Work out the finished part from the listing and answer in its coordinate system (mm). Coordinates: 2 decimals unless noted, no trailing zeros. Answer as a JSON object with one key per item and string values. Group by question number.
1) Each of these flat-tipped pins is pushed along its axis until it touches: P1, Ø4, axis at x = 5.5, y = 13.5, coming from the +Z side; P2, Ø4.5, axis at x = 3, y = 8.5, coming from the +Z side; P3, Ø2, axis at x = 2.5, z = 14, coming from the -Y side. Where does it stop, or does it pass through?
2) Find the intervals of material crossed by line 1 along Y through (x, z) = (1.5, 6.5); line 2 along Z through (x, y) = (3, -7.5); line 3 along Y through (x, z) = (9, 8), in increasing order.
3) Section A-A (x = 9) is taken. Count the separate pieces of the cut face and the enclosed holes in it, plus the area to 3 significant figures.
from build123d import *

# Parameters (mm, degrees)
CUT_EXTRUDE2_DEPTH      = 30.467269979
FILLET1_R               = 0.75
CUT_EXTRUDE3_DEPTH      = 30.467269979
CUT_EXTRUDE3_DEPTH_BACK = 30.467269979
SKETCH2_R               = 1.5


with BuildPart() as part:
    # Sketch1 → Revolve2 (revolve)
    with BuildSketch(Plane.XY, mode=Mode.PRIVATE) as revolve2_sk:
        with BuildLine():
            Line((0, 0), (10, 0))
            Line((10, 0), (10, 19.6))
            Line((10, 19.6), (8.5, 19.6))
            ThreePointArc((8.5, 19.6), (5, 18.170714214), (1.5, 19.6))
            Line((1.5, 19.6), (0, 19.6))
            Line((0, 19.6), (0, 0))
        make_face()
    revolve(revolve2_sk.sketch.rotate(Axis((0, 0, 0), (1, 0, 0)), 90), axis=Axis((0, 0, 0), (1, 0, 0)))

    # Sketch3 → Cut-Extrude2 (cut, through all)
    with BuildSketch(Plane(origin=(10, 0, 0), x_dir=(0, 0, -1), z_dir=(1, 0, 0))):
        with BuildLine():
            Line((2.604722665, 14.772116295), (0.84225046, 4.776639722))
            ThreePointArc((0.84225046, 4.776639722), (1.566792192, 4.590297931), (2.25405939, 4.294751347))
            Line((2.25405939, 4.294751347), (6.970847581, 13.281840385))
            ThreePointArc((6.970847581, 13.281840385), (4.845422268, 14.195840343), (2.604722665, 14.772116295))
        make_face()
        with BuildLine():
            Line((9.171312121, 11.869584406), (2.965590908, 3.838091119))
            ThreePointArc((2.965590908, 3.838091119), (3.520543403, 3.336382325), (3.991740938, 2.755299829))
            Line((3.991740938, 2.755299829), (12.344757988, 8.520971201))
            ThreePointArc((12.344757988, 8.520971201), (10.887544298, 10.318012365), (9.171312121, 11.869584406))
        make_face()
        with BuildLine():
            Line((13.636864497, 6.247873773), (4.409550218, 2.020282094))
            ThreePointArc((4.409550218, 2.020282094), (4.667780547, 1.318141736), (4.814962743, 0.584642325))
            Line((4.814962743, 0.584642325), (14.890633111, 1.808050204))
            ThreePointArc((14.890633111, 1.808050204), (14.435461139, 4.076452099), (13.636864497, 6.247873773))
        make_face()
        with BuildLine():
            Line((14.978375558, -0.805149446), (4.843334715, -0.260349211))
            ThreePointArc((4.843334715, -0.260349211), (4.74568542, -1.002069239), (4.53513461, -1.719949689))
            Line((4.53513461, -1.719949689), (14.02524364, -5.319073306))
            ThreePointArc((14.02524364, -5.319073306), (14.676387798, -3.098974216), (14.978375558, -0.805149446))
        make_face()
        with BuildLine():
            Line((12.888521288, -7.67372263), (4.167569596, -2.48133765))
            ThreePointArc((4.167569596, -2.48133765), (3.736410956, -3.092718228), (3.216361792, -3.630521958))
            Line((3.216361792, -3.630521958), (9.946839874, -11.227661223))
            ThreePointArc((9.946839874, -11.227661223), (11.555130883, -9.564462885), (12.888521288, -7.67372263))
        make_face()
        with BuildLine():
            Line((7.846062115, -12.784338438), (2.537064508, -4.133881536))
            ThreePointArc((2.537064508, -4.133881536), (1.87116977, -4.474862742), (1.160759249, -4.709385399))
            Line((1.160759249, -4.709385399), (3.589734964, -14.564127261))
            ThreePointArc((3.589734964, -14.564127261), (5.786732737, -13.838848371), (7.846062115, -12.784338438))
        make_face()
        with BuildLine():
            ThreePointArc((0.325348516, -4.839402981), (-0.42273386, -4.83187013), (-1.160759249, -4.709385399))
            Line((-1.160759249, -4.709385399), (-3.589734964, -14.564127261))
            ThreePointArc((-3.589734964, -14.564127261), (-1.307336141, -14.942920471), (1.006164666, -14.966216378))
            Line((1.006164666, -14.966216378), (0.325348516, -4.839402981))
        make_face()
        with BuildLine():
            ThreePointArc((-1.9609009, -4.436275524), (-2.619794257, -4.081954301), (-3.216361792, -3.630521958))
            Line((-3.216361792, -3.630521958), (-9.946839874, -11.227661223))
            ThreePointArc((-9.946839874, -11.227661223), (-8.101910065, -12.623749574), (-6.064232982, -13.719514508))
            Line((-6.064232982, -13.719514508), (-1.9609009, -4.436275524))
        make_face()
        with BuildLine():
            ThreePointArc((-3.797931552, -3.016850808), (-4.216691362, -2.396911935), (-4.53513461, -1.719949689))
            Line((-4.53513461, -1.719949689), (-14.02524364, -5.319073306))
            ThreePointArc((-14.02524364, -5.319073306), (-13.040434031, -7.412629781), (-11.745387936, -9.329837203))
            Line((-11.745387936, -9.329837203), (-3.797931552, -3.016850808))
        make_face()
        with BuildLine():
            ThreePointArc((-4.764901855, -0.906301928), (-4.847595293, -0.162765931), (-4.814962743, 0.584642325))
            Line((-4.814962743, 0.584642325), (-14.890633111, 1.808050204))
            ThreePointArc((-14.890633111, 1.808050204), (-14.991551715, -0.503365838), (-14.735816061, -2.802806631))
            Line((-14.735816061, -2.802806631), (-4.764901855, -0.906301928))
        make_face()
        with BuildLine():
            ThreePointArc((-4.640290566, 1.411869801), (-4.367973561, 2.108667787), (-3.991740938, 2.755299829))
            Line((-3.991740938, 2.755299829), (-12.344757988, 8.520971201))
            ThreePointArc((-12.344757988, 8.520971201), (-13.508285569, 6.521213153), (-14.350446312, 4.366313163))
            Line((-14.350446312, 4.366313163), (-4.640290566, 1.411869801))
        make_face()
        with BuildLine():
            ThreePointArc((-3.45264463, 3.406599173), (-2.887701727, 3.897031127), (-2.25405939, 4.294751347))
            Line((-2.25405939, 4.294751347), (-6.970847581, 13.281840385))
            ThreePointArc((-6.970847581, 13.281840385), (-8.930433992, 12.051860799), (-10.677562255, 10.53516323))
            Line((-10.677562255, 10.53516323), (-3.45264463, 3.406599173))
        make_face()
        with BuildLine():
            ThreePointArc((-1.474039418, 4.620917729), (-0.745892228, 4.7926316), (0, 4.850327089))
            Line((0, 4.850327089), (0, 15))
            ThreePointArc((0, 15), (-2.30672761, 14.821572377), (-4.558577364, 14.290534364))
            Line((-4.558577364, 14.290534364), (-1.474039418, 4.620917729))
        make_face()
    extrude(amount=-CUT_EXTRUDE2_DEPTH, mode=Mode.SUBTRACT)

    # Fillet1
    fillet1_edges = [part.edges().sort_by_distance(p)[0] for p in [
        (5, -11.227661223, -9.946839874),
        (5, 2.755299829, -3.991740938),
        (5, 3.838091119, -2.965590908),
        (5, 11.869584406, -9.171312121),
        (5, 8.520971201, -12.344757988),
        (5, 0.584642325, -4.814962743),
        (5, 2.020282094, -4.409550218),
        (5, 6.247873773, -13.636864497),
        (5, 1.808050204, -14.890633111),
        (5, 4.294751347, 2.25405939),
        (5, 3.406599173, 3.45264463),
        (5, 10.53516323, 10.677562255),
        (5, 13.281840385, 6.970847581),
        (5, 4.850327089, 0),
        (5, 4.620917729, 1.474039418),
        (5, 14.290534364, 4.558577364),
        (5, 15, 0),
        (5, 0.584642325, 4.814962743),
        (5, -0.906301928, 4.764901855),
        (5, -2.802806631, 14.735816061),
        (5, 1.808050204, 14.890633111),
        (5, 2.755299829, 3.991740938),
        (5, 1.411869801, 4.640290566),
        (5, 4.366313163, 14.350446312),
        (5, 8.520971201, 12.344757988),
        (5, 4.294751347, -2.25405939),
        (5, 4.776639722, -0.84225046),
        (5, 14.772116295, -2.604722665),
        (5, 13.281840385, -6.970847581),
        (5, -4.709385399, -1.160759249),
        (5, -4.133881536, -2.537064508),
        (5, -12.784338438, -7.846062115),
        (5, -14.564127261, -3.589734964),
        (5, -4.709385399, 1.160759249),
        (5, -4.839402981, -0.325348516),
        (5, -14.966216378, -1.006164666),
        (5, -14.564127261, 3.589734964),
        (5, -1.719949689, 4.53513461),
        (5, -3.016850808, 3.797931552),
        (5, -9.329837203, 11.745387936),
        (5, -5.319073306, 14.02524364),
        (5, -3.630521958, 3.216361792),
        (5, -4.436275524, 1.9609009),
        (5, -13.719514508, 6.064232982),
        (5, -11.227661223, 9.946839874),
        (5, -1.719949689, -4.53513461),
        (5, -0.260349211, -4.843334715),
        (5, -0.805149446, -14.978375558),
        (5, -5.319073306, -14.02524364),
        (5, -3.630521958, -3.216361792),
        (5, -2.48133765, -4.167569596),
        (5, -7.67372263, -12.888521288),
    ]]
    fillet(fillet1_edges, radius=FILLET1_R)

    # Sketch2 → Cut-Extrude3 (cut, two sides: drawn at the far end of the back side and taken through both)
    with BuildSketch(Plane(origin=(10, 0, 0), x_dir=(0, 0, -1), z_dir=(1, 0, 0)).offset(-CUT_EXTRUDE3_DEPTH_BACK)):
        Circle(SKETCH2_R)
    extrude(amount=CUT_EXTRUDE3_DEPTH + CUT_EXTRUDE3_DEPTH_BACK, mode=Mode.SUBTRACT)


solid = part.part
Report:
{
 "1": {"P1": "stops at z = 14.15", "P2": "stops at z = 18.37", "P3": "stops at y = -14.05"},
 "2": {"line 1": "y = -18.49 to -13.46, -7.34 to -5.16, -2.47 to -1.24, 0.79 to 1.98, 4.49 to 6.41, 12.38 to 18.49", "line 2": "z = -17.01 to -12.46, -6.64 to -4.6, -1.85 to -0.5, 1.85 to 3.32, 6.64 to 9.44, 12.99 to 17.01", "line 3": "y = -17.89 to -12.69, -9.03 to -6.35, -3.03 to -1.52, 0.97 to 2.43, 5.52 to 7.89, 12.69 to 17.89"},
 "3": {"separate pieces": "1", "enclosed holes": "14", "area": "801 mm²"}
}
